Source: three-view drawing plus pictorial views. Frame: mm from the lowest corner of the part. Give positions to 0.01 mm unless a question says otherwise; leave off trailing zeros. Order: outer loops, then holes, each group sorted by start corner. A loop starts at its lowest first (then second) coordinate and runs counter-clockwise, first axis right, second up. Notation, with made-up numbers: M 86.25,-1 L 120.25,-1 A22 cw 120.25,15 Z; hole C 89.25,-29 d5. An arc over 180 degrees is marked long. Use CSV: the item, a comma, the result in double quotes. Start each with the question number.
1. Section query A-A, the plane x = 5. Return the cut outline in (y, z), plus the area to 3 significant figures.
2. Section query B-B, the plane y = 36. Return the cut outline in (x, z).
3. Pin query (flat end, axial travel): P1, Ø1.5, axis at y = 50, z = 2, coming from the -X side; P2, Ø1.5, axis at y = 47, z = 2, coming from the +X side; P3, Ø1.5, axis at x = 12.5, z = 1.5, coming from the +Y side. Return the tip coordinate at first contact, or that it passes through.
4. Line query: line 1 along X through (y, z) = (31, 1.7); line 2 along X through (y, z) = (6.5, 2.4); line 3 along Y through (x, z) = (5, 0.75). Output: solid intervals per line, ascending. Write a range as [from, to].
5. Section query D-D, the plane y = 51. Return the cut outline in (x, z), plus the area to 3 significant figures.
6. Section query C-C, the plane z = 0.45. Return the cut outline in (x, y).
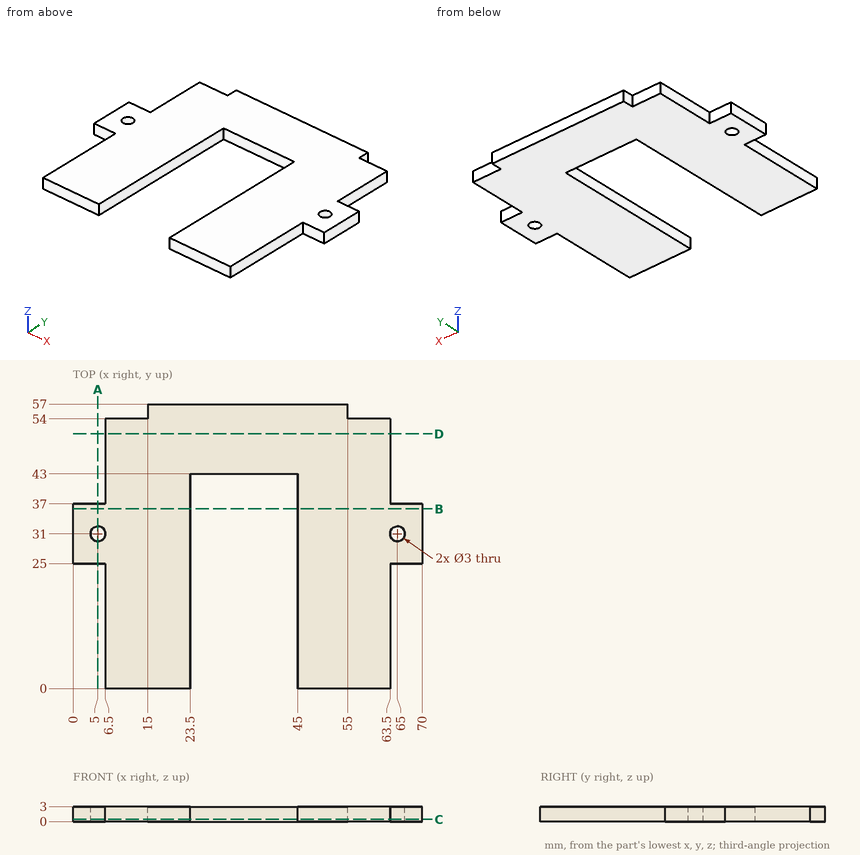
Result set:
1,outline,"M 25,0 L 29.5,0 L 29.5,3 L 25,3 Z; M 32.5,0 L 37,0 L 37,3 L 32.5,3 Z"
1,area,"27.0 mm2"
2,outline,"M 0,0 L 23.5,0 L 23.5,3 L 0,3 Z; M 45,0 L 70,0 L 70,3 L 45,3 Z"
3,P1,"x = 6.5"
3,P2,"x = 63.5"
3,P3,"y = 54"
4,line 1,"[0, 3.5], [6.5, 23.5], [45, 63.5], [66.5, 70]"
4,line 2,"[6.5, 23.5], [45, 63.5]"
4,line 3,"[25, 29.5], [32.5, 37]"
5,outline,"M 6.5,0 L 63.5,0 L 63.5,3 L 6.5,3 Z"
5,area,"171 mm2"
6,outline,"M 0,25 L 6.5,25 L 6.5,0 L 23.5,0 L 23.5,43 L 45,43 L 45,0 L 63.5,0 L 63.5,25 L 70,25 L 70,37 L 63.5,37 L 63.5,54 L 55,54 L 55,57 L 15,57 L 15,54 L 6.5,54 L 6.5,37 L 0,37 Z; hole C 5,31 d3; hole C 65,31 d3"
